The model under review builds one solid part; all positions refer to its coordinate system, in mm. Face numbers are marked on the shaded views. Round coordinates to 2 decimals unless told otherwise and drop trailing zeros. Order: outer loops, then holes, each group sorted by start corner. A loop starts at its lowest first (then second) coordinate and runs counter-clockwise, first axis right, second up. Notation, with made-up numbers: M 24,2 L 44,2 A23 cw 44,18 Z; hole C 61.5,-5 d5. An arc over 180 degrees is marked long. Use a Markdown table: item, result. Add a question column.
1. Consider section B-B on y = 20. State the section outline as (x, z) points, then the cut area to 3 significant figures.
2. Insertion check: P1, Ø12, axis at x = -45, z = 15.5, coming from the +Y side; P2, Ø3, axis at x = -8.5, z = 35.5, coming from the +Y side; P3, Ø11.5, axis at x = 45, y = 55, coming from the -Z side; P4, Ø10, axis at x = -24.5, z = 28.5, coming from the -Y side. Each pin has a flat end and moves straight along its axis. Give the tip position at first contact, or say it passes through.
3. Consider section D-D on z = 56.5. State the section outline as (x, y) points.
4. Consider section A-A on x = 0. State the section outline as (y, z) points.
5. Consider section C-C on y = 55. State the section outline as (x, z) points.
6. The part is to be moulded in two halves that separate along Y. For the marked faces 1, 2 and 3, say which applies: +Y half, -Y half, draft (parallel to the pull), parting line (faces both ways), or undercut.
7. To check wall thickness, follow probe 1 along X at (y, z) = (55, 4.75); probe 2 along Y at (x, z) = (0, 4); probe 3 along X at (y, z) = (20, 51). State the ranges of each line that lie inside material, in increasing order.
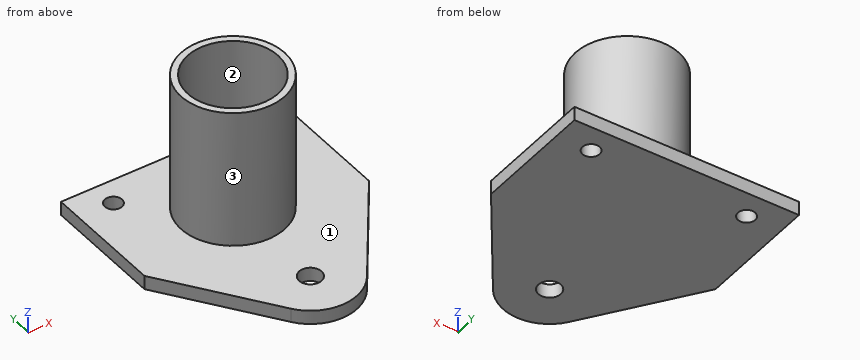
Autodesk Inventor part; units mm, degrees
ref_plane "YZ Plane" through (0, 0, 0) normal (1, 0, 0) x (0, 1, 0)
ref_plane "XZ Plane" through (0, 0, 0) normal (0, 1, 0) x (-1, 0, 0)
ref_plane "XY Plane" through (0, 0, 0) normal (0, 0, 1) x (1, 0, 0)
sketch "Boceto1" plane through (0, 0, 0) normal (0, 0, 1) x (1, 0, 0)
  line L0 (0, 0) -> (0, 40)
  line L1 (65, 70) -> (-65, 70)
  line L2 (-65, 70) -> (-65, 10)
  line L3 (-65, 10) -> (65, 10)
  line L4 (65, 10) -> (65, 70)
  line L5 (65, 70) -> (-65, 10) construction
  line L6 (-65, 70) -> (65, 10) construction
  line L7 (65, 70) -> (-65, 70)
  line L8 (-65, 70) -> (-65, 0)
  line L9 (65, 0) -> (65, 70)
  line L10 (65, 70) -> (65, 40)
  line L11 (65, 55) -> (-65, 55)
  line L12 (65, 55) -> (45, 55)
  circle A0 centre (45, 55) radius 5
  line L13 (-65, 55) -> (-62.9791, 55)
  line L14 (-65, 55) -> (-45, 55)
  circle A1 centre (-45, 55) radius 5
  line L15 (6.5, -45) -> (-6.5, -45)
  circle A2 centre (0, -45) radius 6.5
  arc A3 (-22.0262, -60.6156) -> (22.0262, -60.6156) centre (0, -45) ccw
  line L16 (65, 0) -> (22.0262, -60.6156)
  line L17 (-65, 0) -> (-22.0262, -60.6156)
  dimension "d0" = 130
  dimension "d1" = 60
  dimension "d2" = 20
  dimension "d3" = 10
  dimension "d4" = 20
  dimension "d5" = 10
  dimension "d6" = 13
extrude "Extrusión1" add sketch "Boceto1" along normal blind 8 contours L4 L11 A0 A1 L2 L1 | L4 L3 L2 L11 A1 A0 | L3 L9 L16 A3 L17 L8
sketch "Boceto2" plane through (0, 0, 8) normal (0, 0, 1) x (1, 0, 0)
  line L0 (65, 70) -> (-65, 70)
  line L1 (-65, 70) -> (-65, 40)
  line L2 (-65, 70) -> (-65, 0)
  line L3 (65, 0) -> (65, 70)
  line L4 (-65, 70) -> (-65, 50)
  line L5 (-65, 50) -> (65, 50)
  line L6 (-65, 50) -> (-65, -30)
  line L7 (-65, -30) -> (65, -30)
  line L8 (0, 50) -> (0, -30)
  line L9 (0, 10) -> (0, 20)
  circle A0 centre (0, 20) radius 30
  circle A1 centre (0, 20) radius 26.15
  point P0 (0, 0)
  dimension "d13" = 30
  dimension "d15" = 20
  dimension "d16" = 80
  dimension "d23" = 10
  dimension "d24" = 52.3
extrude "Extrusión4" add sketch "Boceto2" along normal blind 80 contours A0 L8 A1 | L8 A1 A0
properties part number "encaje"
Answer block:
| question | item | result |
|---|---|---|
| 1 | outline | M -65,0 L 65,0 L 65,8 L 30,8 L 30,88 L 26.15,88 L 26.15,8 L -26.15,8 L -26.15,88 L -30,88 L -30,8 L -65,8 Z |
| 1 | area | 1,660 mm^2 |
| 2 | P1 | through |
| 2 | P2 | y = 49.17 |
| 2 | P3 | z = 0 |
| 2 | P4 | y = -2.8 |
| 3 | outline | C 0,20 d60; hole C 0,20 d52.3 |
| 4 | outline | M -72,0 L -51.5,0 L -51.5,8 L -72,8 Z; M -38.5,0 L 70,0 L 70,8 L 50,8 L 50,88 L 46.15,88 L 46.15,8 L -6.15,8 L -6.15,88 L -10,88 L -10,8 L -38.5,8 Z |
| 5 | outline | M -65,0 L -50,0 L -50,8 L -65,8 Z; M -40,0 L 40,0 L 40,8 L -40,8 Z; M 50,0 L 65,0 L 65,8 L 50,8 Z |
| 6 | face 1 | draft |
| 6 | face 2 | undercut |
| 6 | face 3 | parting line |
| 7 | probe 1 | -65 to -50, -40 to 40, 50 to 65 |
| 7 | probe 2 | -72 to -51.5, -38.5 to 70 |
| 7 | probe 3 | -30 to -26.15, 26.15 to 30 |
